The listing builds one solid part. Answer for the finished solid, in the listing's coordinates (mm). A direction names the side the tool comes from. Give positions to 0.01 mm unless a question says otherwise; leave off trailing zeros. Order: outer loops, then holes, each group sorted by start corner. A loop starts at its lowest first (then second) coordinate and runs counter-clockwise, first axis right, second up.
```python
from build123d import *

# Parameters (mm, degrees)
THICKNESS_T   = 2
SKETCH001_R   = 6.5
SKETCH001_R_2 = 4
PAD_DEPTH     = 250


with BuildPart() as part:
    # Sketch → Revolution (revolve)
    with BuildSketch(Plane.XZ):
        Polygon((0, 0), (8, 0), (4, 5), (0, 5), align=None)
    revolve(axis=Axis((0, 0, 0), (0, 0, 1)))

    # Thickness
    thickness_openings = [part.faces().sort_by_distance(p)[0] for p in [
        (0, 0, 5),
        (0, 0, 0),
    ]]
    offset(amount=THICKNESS_T, openings=thickness_openings)

    # Sketch001 (on Face4 of Thickness) → Pad (new body)
    with BuildSketch(Plane.XY.offset(5)):
        Circle(SKETCH001_R)
        Circle(SKETCH001_R_2, mode=Mode.SUBTRACT)
    extrude(amount=PAD_DEPTH)


solid = part.part
```
1) For a pull along Y with two mould halves and no side action, classify faces 1 (the flat face through (3, 3, 255)), 2 (the cylindrical face through (-0.867, -3.905, 128.25)), 3 (the conical face through (-1.464, -6.595, 4.757)) as +Y half, -Y half, draft (parallel to the pull), parting line (faces both ways), or undercut.
Geometry says:
face 1: draft
face 2: undercut
face 3: parting line
2) A tool of negligible diameter and unlimited length cuts with its end or side. For faces 4 (the cylindrical face through (-5.158, -3.955, 128.25)), 5 (the flat face through (2, 8, 0)), from which of +Z, -Z, +X, -X, +Y, -Y can it reach the whole face along a straight path? Write none if from no direction.
Geometry says:
face 4: +Z
face 5: -Z, +X, -X, +Y, -Y
3) Given P1, Ø10, axis at x = 8.5, y = -1, coming from the +Z side; P2, Ø4, axis at x = -1, z = 142, coming from the +Y side; P3, Ø4, axis at y = -2.5, z = 220.5, coming from the -X side; P4, Ø1.5, axis at x = -2, y = -1, coming from the -Z side, each flat-ended and moving along its own axis, determine where each tip first touches the part or whether it passes through.
Geometry says:
P1: stops at z = 255
P2: stops at y = 6.5
P3: stops at x = -6.48
P4: passes through
4) Straight lines are drawn through the part: probe 1 along Y at (x, z) = (1.75, 139.5); probe 2 along X at (y, z) = (0.75, 98); probe 3 along Y at (x, z) = (0, 118). For each, find the intervals that lie inside material, in ascending order.
Geometry says:
probe 1: y = -6.26 to -3.6, 3.6 to 6.26
probe 2: x = -6.46 to -3.93, 3.93 to 6.46
probe 3: y = -6.5 to -4, 4 to 6.5
5) Find section C-C (z = 103). Write down the section's boundary in (x, y), then the cut area to 3 significant figures.
Geometry says:
outline: circle Ø13 at (0, 0); hole circle Ø8 at (0, 0)
area: 82.5 mm2
6) Find section A-A (x = 0). Write down the section's boundary in (y, z).
Geometry says:
outline: (-10.56, 0) - (-8, 0) - (-4, 5) - (-4, 255) - (-6.5, 255) - (-6.5, 5) - (-6.56, 5) - close; (4, 5) - (8, 0) - (10.56, 0) - (6.56, 5) - (6.5, 5) - (6.5, 255) - (4, 255) - close
